```python
from build123d import *

# Parameters (mm, degrees)
SKETCH039_R             = 2.25
PAD020_DEPTH            = 5
FILLET008_R             = 9
CHAMFER018_SIZE         = 3
SKETCH047_R             = 2.1
POCKET026_DEPTH         = 5.001
BODY013_PLACEMENT_ANGLE = 180


with BuildPart() as part:
    # Sketch039 → Pad020 (new body)
    with BuildSketch(Plane.XY):
        Polygon((100, -10), (100, 70), (140, 70), (140, 100), (127.28, 180), (-5, 180), (-5, 115), (5, 115), (5, 50), (18, 50), (40, 10), (40, -10), align=None)
        with Locations((90, 0)):
            Circle(SKETCH039_R, mode=Mode.SUBTRACT)
        with Locations((50, 0)):
            Circle(SKETCH039_R, mode=Mode.SUBTRACT)
        with Locations((0, 125)):
            Circle(SKETCH039_R, mode=Mode.SUBTRACT)
        with Locations((0, 170)):
            Circle(SKETCH039_R, mode=Mode.SUBTRACT)
    extrude(amount=-PAD020_DEPTH)

    # Fillet008
    fillet008_edges = [part.edges().sort_by_distance(p)[0] for p in [
        (100, 70, -2.5),
        (140, 70, -2.5),
    ]]
    fillet(fillet008_edges, radius=FILLET008_R)

    # Chamfer018
    chamfer018_edges = [part.edges().sort_by_distance(p)[0] for p in [
        (-5, 115, -2.5),
        (5, 50, -2.5),
        (-5, 180, -2.5),
        (127.28, 180, -2.5),
        (100, -10, -2.5),
        (40, -10, -2.5),
    ]]
    chamfer(chamfer018_edges, length=CHAMFER018_SIZE)

    # Sketch047 (on Face2 of Chamfer018) → Pocket026 (cut, through all)
    with BuildSketch(Plane.XY):
        with Locations((120.793214, 169.850903)):
            Circle(SKETCH047_R)
        with Locations((131, 79)):
            Circle(SKETCH047_R)
        with Locations((131, 105.657278)):
            Circle(SKETCH047_R)
        with BuildLine():
            ThreePointArc((27.5, 80), (25, 82.5), (22.5, 80))
            Line((22.5, 80), (22.5, 60))
            ThreePointArc((22.5, 60), (25, 57.5), (27.5, 60))
            Line((27.5, 60), (27.5, 80))
        make_face()
        with BuildLine():
            ThreePointArc((87.5, 80), (85, 82.5), (82.5, 80))
            Line((82.5, 80), (82.5, 60))
            ThreePointArc((82.5, 60), (85, 57.5), (87.5, 60))
            Line((87.5, 60), (87.5, 80))
        make_face()
        with BuildLine():
            ThreePointArc((27.5, 140), (25, 142.5), (22.5, 140))
            Line((22.5, 140), (22.5, 120))
            ThreePointArc((22.5, 120), (25, 117.5), (27.5, 120))
            Line((27.5, 120), (27.5, 140))
        make_face()
        with BuildLine():
            ThreePointArc((87.5, 140), (85, 142.5), (82.5, 140))
            Line((82.5, 140), (82.5, 120))
            ThreePointArc((82.5, 120), (85, 117.5), (87.5, 120))
            Line((87.5, 120), (87.5, 140))
        make_face()
    extrude(amount=-POCKET026_DEPTH, mode=Mode.SUBTRACT)


with BuildPart() as part_1:
    # Body013 placement: moved
    add(part.part.moved(Location((0, 0, -42.3))).rotate(Axis((0, 0, -42.3), (0, 1, 0)), BODY013_PLACEMENT_ANGLE))


solid = part_1.part
```
Check sheet for the modelled part. Datum: model origin and axes. Units: mm. A direction names the side the tool comes from. Give positions to 0.01 mm unless a question says otherwise; leave off trailing zeros. Loops run counter-clockwise (first coordinate to the right, second up) from the corner with the lowest first, then second, coordinate; pieces in that order, holes last. Notation, with made-up numbers: M 2.25,27 L 47.25,27 A15 ccw 47.25,41 Z; hole C -33.5,46 d6. An arc over 180 degrees is marked long. Answer in a Markdown table with one row per item.
1) Cross-section at D-D (y = 85.5). Enter the section's corners in (x, z), plus the area to 3 significant figures.
Solutions:
| item | result |
|---|---|
| outline | M -140,-42.3 L -5,-42.3 L -5,-37.3 L -140,-37.3 Z |
| area | 675 mm^2 |
2) Depth check by flat-ended pin: pin 1 (2.5 mm diameter, centred on y = 5.5, z = -39, fed in from +X); pin 2 (1 mm diameter, centred on y = 62, z = -41.5, fed in from -X); pin 3 (2.5 mm diameter, centred on x = -0.5, z = -39.5, fed in from -Y). Enter the tip coordinate at first touch or a pass-through.
Solutions:
| item | result |
|---|---|
| pin 1 | stops at x = -40 |
| pin 2 | stops at x = -100.13 |
| pin 3 | stops at y = 115 |
3) Cross-section at A-A (x = 0). Enter the section's corners in (y, z).
Solutions:
| item | result |
|---|---|
| outline | M 115,-42.3 L 122.75,-42.3 L 122.75,-37.3 L 115,-37.3 Z; M 127.25,-42.3 L 167.75,-42.3 L 167.75,-37.3 L 127.25,-37.3 Z; M 172.25,-42.3 L 180,-42.3 L 180,-37.3 L 172.25,-37.3 Z |
4) Tool access check on faces 1 (the face through (-1, 115, -40)), 2 (the face through (-82.5, 70, -40)), 3 (the face through (-102.566, 67.294, -39.765)). Record the directions out of +Z, -Z, +X, -X, +Y, -Y that give a thin tool (end or side, any length) a straight path to the whole face; none if there is none.
Solutions:
| item | result |
|---|---|
| face 1 | +Z, -Z, +X, -Y |
| face 2 | +Z, -Z |
| face 3 | +Z, -Z, -X, -Y |
5) Mould release check, pull along Y, two halves, no side actions. Record for faces 4 (the face through (-47.752, 0.099, -39.835)), 5 (the face through (-137.294, 72.566, -39.765)), 6 (the face through (-140, 89, -40)): released by +Y, released by -Y, zero draft, split by the parting line, or undercut.
Solutions:
| item | result |
|---|---|
| face 4 | undercut |
| face 5 | released by -Y |
| face 6 | zero draft |
6) Cross-section at B-B (x = -50). Enter the section's corners in (y, z).
Solutions:
| item | result |
|---|---|
| outline | M -10,-42.3 L -2.25,-42.3 L -2.25,-37.3 L -10,-37.3 Z; M 2.25,-42.3 L 180,-42.3 L 180,-37.3 L 2.25,-37.3 Z |
7) Thickness scan on line 1 (Y direction, x = 0, z = -40.8); line 2 (X direction, y = 170, z = -39.6); line 3 (X direction, y = 61.5, z = -41.95). Record the ranges inside material, lowest first.
Solutions:
| item | result |
|---|---|
| line 1 | y = 115 to 122.75, 127.25 to 167.75, 172.25 to 180 |
| line 2 | x = -128.87 to -122.89, -118.7 to -2.25, 2.25 to 5 |
| line 3 | x = -100.01 to -87.5, -82.5 to -27.5, -22.5 to -5 |
8) Cross-section at C-C (y = 65). Enter the section's corners in (x, z), plus the area to 3 significant figures.
Solutions:
| item | result |
|---|---|
| outline | M -100.94,-42.3 L -87.5,-42.3 L -87.5,-37.3 L -100.94,-37.3 Z; M -82.5,-42.3 L -27.5,-42.3 L -27.5,-37.3 L -82.5,-37.3 Z; M -22.5,-42.3 L -5,-42.3 L -5,-37.3 L -22.5,-37.3 Z |
| area | 430 mm^2 |
